```python
from build123d import *

# Parameters (mm, degrees)
SKETCH4_R           = 10.6
BOSS_EXTRUDE3_DEPTH = 15
SKETCH5_R           = 1.5
CUT_EXTRUDE2_DEPTH  = 15
SKETCH4_2_R         = 10.6
BOSS_EXTRUDE4_DEPTH = 8


with BuildPart() as part:
    # Sketch4 → Boss-Extrude3 (new body)
    with BuildSketch(Plane.XY):
        with BuildLine():
            Line((-59, -30.1), (59, -30.1))
            Line((59, -30.1), (59, -22.100006907))
            Line((59, -22.100006907), (47.694750419, -22.100006907))
            ThreePointArc((47.694750419, -22.100006907), (38.263703272, -19.736768223), (31.061437671, -13.20554188))
            Line((31.061437671, -13.20554188), (15.385814292, 10.27261985))
            ThreePointArc((15.385814292, 10.27261985), (0, 18.5), (-15.385814292, 10.27261985))
            Line((-15.385814292, 10.27261985), (-31.061437671, -13.20554188))
            ThreePointArc((-31.061437671, -13.20554188), (-38.263703272, -19.736768223), (-47.694750419, -22.100006907))
            Line((-47.694750419, -22.100006907), (-59, -22.100006907))
            Line((-59, -22.100006907), (-59, -30.1))
        make_face()
        Circle(SKETCH4_R, mode=Mode.SUBTRACT)
    extrude(amount=BOSS_EXTRUDE3_DEPTH)

    # Sketch5 → Cut-Extrude2 (cut)
    with BuildSketch(Plane.XZ.offset(30.1)):
        with Locations((50, 7.5)):
            Circle(SKETCH5_R)
        with Locations((-50, 7.5)):
            Circle(SKETCH5_R)
    extrude(amount=-CUT_EXTRUDE2_DEPTH, mode=Mode.SUBTRACT)

    # Sketch4<2> → Boss-Extrude4 (add)
    with BuildSketch(Plane.XY):
        Circle(SKETCH4_2_R)
    extrude(amount=BOSS_EXTRUDE4_DEPTH)


solid = part.part
```
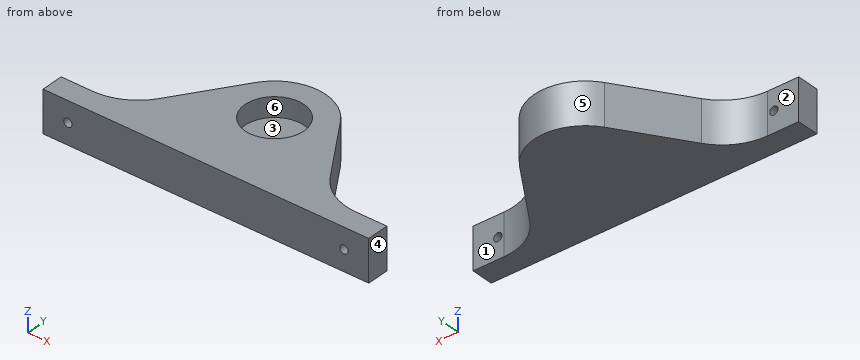
Geometry check sheet. Reference: the model listing, model coordinates, mm. Face numbers are marked on the shaded views. A direction names the side the tool comes from. Round coordinates to 2 decimals unless told otherwise and drop trailing zeros. Order: outer loops, then holes, each group sorted by start corner. A loop starts at its lowest first (then second) coordinate and runs counter-clockwise, first axis right, second up. Notation, with made-up numbers: (-5, -27.5) -> (51, -27.5) arc R29 ccw to (51, -0.5) -> close; hole circle Ø7 at (33.25, -10.75). An arc over 180 degrees is marked (long way). Return JSON: item names as keys, results as strings. Group by question number.
Q1. Section check B-B, the plane y = 0. Record the boundary of the cut face in (x, z).
Q2. Section check A-A, the plane x = -50. Record the boundary of the cut face in (y, z).
Q3. Section check D-D, the plane y = 14. Record the boundary of the cut face in (x, z), plus the area to 3 significant figures.
Q4. Gauge pin test, flat ends, axial feed: pin 1 (3.5 mm diameter, centred on x = -55.5, z = 8, fed in from +Y); pin 2 (1.5 mm diameter, centred on x = 20.5, z = 3, fed in from +Y); pin 3 (2 mm diameter, centred on x = 42.5, y = -21, fed in from +Z); pin 4 (17 mm diameter, centred on x = 0.5, y = 0.5, fed in from +Z). Record the tip position at first contact, or that the pin passes through.
Q5. Release check for a two-part mould opening along X. For the marked faces 4, 5 and 6 record: released by +X, released by -X, zero draft, split by the parting line, or undercut.
Q6. Material ranges on probe 1 along Z at (x, y) = (50, -28); probe 2 along X at (y, z) = (-26, 7.75); probe 3 along Y at (x, z) = (0, 10.25), recorded low to high. Write a range as from..to.
Q7. Section check C-C, the plane x = -1.5. Record the boundary of the cut face in (y, z).
Q8. Tool access check on the marked faces 1, 2 and 3. Record the directions out of +Z, -Z, +X, -X, +Y, -Y that give a thin tool (end or side, any length) a straight path to the whole face; none if there is none.
Numbers:
{
 "1": {"outline": "(-22.24, 0) -> (22.24, 0) -> (22.24, 15) -> (10.6, 15) -> (10.6, 8) -> (-10.6, 8) -> (-10.6, 15) -> (-22.24, 15) -> close"},
 "2": {"outline": "(-30.1, 0) -> (-22.1, 0) -> (-22.1, 6) -> (-30.1, 6) -> close; (-30.1, 9) -> (-22.1, 9) -> (-22.1, 15) -> (-30.1, 15) -> close"},
 "3": {"outline": "(-12.09, 0) -> (12.09, 0) -> (12.09, 15) -> (-12.09, 15) -> close", "area": "363 mm^2"},
 "4": {"pin 1": "y = -22.1", "pin 2": "y = 3.74", "pin 3": "z = 15", "pin 4": "z = 8"},
 "5": {"face 4": "released by +X", "face 5": "split by the parting line", "face 6": "undercut"},
 "6": {"probe 1": "0..6, 9..15", "probe 2": "-59..-51.48, -48.52..48.52, 51.48..59", "probe 3": "-30.1..-10.6, 10.6..18.5"},
 "7": {"outline": "(-30.1, 0) -> (18.44, 0) -> (18.44, 15) -> (10.49, 15) -> (10.49, 8) -> (-10.49, 8) -> (-10.49, 15) -> (-30.1, 15) -> close"},
 "8": {"face 1": "+Z, -Z, +X, +Y", "face 2": "+Z, -Z, -X, +Y", "face 3": "+Z"}
}
